```python
from build123d import *

# Parameters (mm, degrees)
PAD_DEPTH    = 550
SKETCH001_W  = 677.16
SKETCH001_H  = 560
POCKET_DEPTH = 530


with BuildPart() as part:
    # Sketch → Pad (new body)
    with BuildSketch(Plane.XY):
        Polygon((-500, 300), (500, 300), (500, -300), (-217.157288, -300), (-500, -17.157288), align=None)
    extrude(amount=PAD_DEPTH)

    # Sketch001 → Pocket (cut)
    with BuildSketch(Plane.XY.offset(551)):
        with Locations((141.42, 0)):
            Rectangle(SKETCH001_W, SKETCH001_H)
        Polygon((-480, 280), (-217.16, 280), (-217.16, -270), (-480, -7.16), align=None)
    extrude(amount=-POCKET_DEPTH, mode=Mode.SUBTRACT)


solid = part.part
```
Source: CAD feature listing. Evaluate the final solid. Frame: model axes, mm. A direction names the side the tool comes from. Round coordinates to 2 decimals unless told otherwise and drop trailing zeros. Loops run counter-clockwise (first coordinate to the right, second up) from the corner with the lowest first, then second, coordinate; pieces in that order, holes last.
1. Section query A-A on z = 320.5. Output: boundary loops of the cut face in (x, y), and give its area (3 significant figures).
2. Section query C-C on y = 100.5. Output: boundary loops of the cut face in (x, z).
3. Section query D-D on x = -253. Output: boundary loops of the cut face in (y, z).
4. Access query for faces 1 (the flat face through (-347, 70, 21)), 2 (the flat face through (-356.6, -160.56, 271.15)). Directions: +Z, -Z, +X, -X, +Y, -Y. A direction counts if a zero-diameter tool reaches every point of the face in a straight line with its end or side. Return the directions, or none.
5. Ray query, L1, parallel to X at y = 258, z = 493.5; L2, parallel to Y at x = 402, z = 519.5; L3, parallel to X at y = -237.5, z = 494. Return the intervals inside material, ascending.
6. Mould query, pull axis Y, two halves, no side actions, for faces 3 (the flat face through (7, 4, 0)), 4 (the flat face through (137, -280, 289)), 5 (the flat face through (146, -300, 271)), 6 (the flat face through (-480, 134, 289)). Classes: released by +Y, released by -Y, zero draft, split by the parting line, or undercut.
7. Contact query for flat-ended pins moving along their axis: pin 1 (5 mm diameter, centred on x = -98.5, y = -33.5, fed in from -Z); pin 2 (1 mm diameter, centred on x = -121.5, y = 39.5, fed in from +Z). Output: stop coordinate, or through.
8. Section query B-B on x = 10. Output: boundary loops of the cut face in (y, z), and give its area (3 significant figures).
Answers below:
1. outline: (-500, -17.16) - (-217.16, -300) - (500, -300) - (500, 300) - (-500, 300) - close; hole (-480, -7.16) - (-217.16, -270) - (-217.16, 280) - (-480, 280) - close; hole (-197.16, -280) - (480, -280) - (480, 280) - (-197.16, 280) - close
1. area: 70,800 mm2
2. outline: (-500, 0) - (500, 0) - (500, 550) - (480, 550) - (480, 21) - (-197.16, 21) - (-197.16, 550) - (-217.16, 550) - (-217.16, 21) - (-480, 21) - (-480, 550) - (-500, 550) - close
3. outline: (-264.16, 0) - (300, 0) - (300, 550) - (280, 550) - (280, 21) - (-234.16, 21) - (-234.16, 550) - (-264.16, 550) - close
4. face 1: +Z
4. face 2: +Z, -Z, -X, -Y
5. L1: x = -500 to -480, -217.16 to -197.16, 480 to 500
5. L2: y = -300 to -280, 280 to 300
5. L3: x = -279.66 to -249.66, -217.16 to -197.16, 480 to 500
6. face 3: zero draft
6. face 4: undercut
6. face 5: released by -Y
6. face 6: undercut
7. pin 1: stops at z = 0
7. pin 2: stops at z = 21
8. outline: (-300, 0) - (300, 0) - (300, 550) - (280, 550) - (280, 21) - (-280, 21) - (-280, 550) - (-300, 550) - close
8. area: 33,800 mm2
